Drawing for the job (mm, zero at the part's lowest x, y, z). Give positions to 0.01 mm unless a question says otherwise; leave off trailing zeros. Order: outer loops, then holes, each group sorted by start corner. A loop starts at its lowest first (then second) coordinate and runs counter-clockwise, first axis right, second up. Notation, with made-up numbers: (-21, -24.5) - (23, -24.5) arc R26 ccw to (23, 2.5) - close; hole circle Ø10 at (81, 19.5). An arc over 180 degrees is marked (long way). One line per item, written item: value.
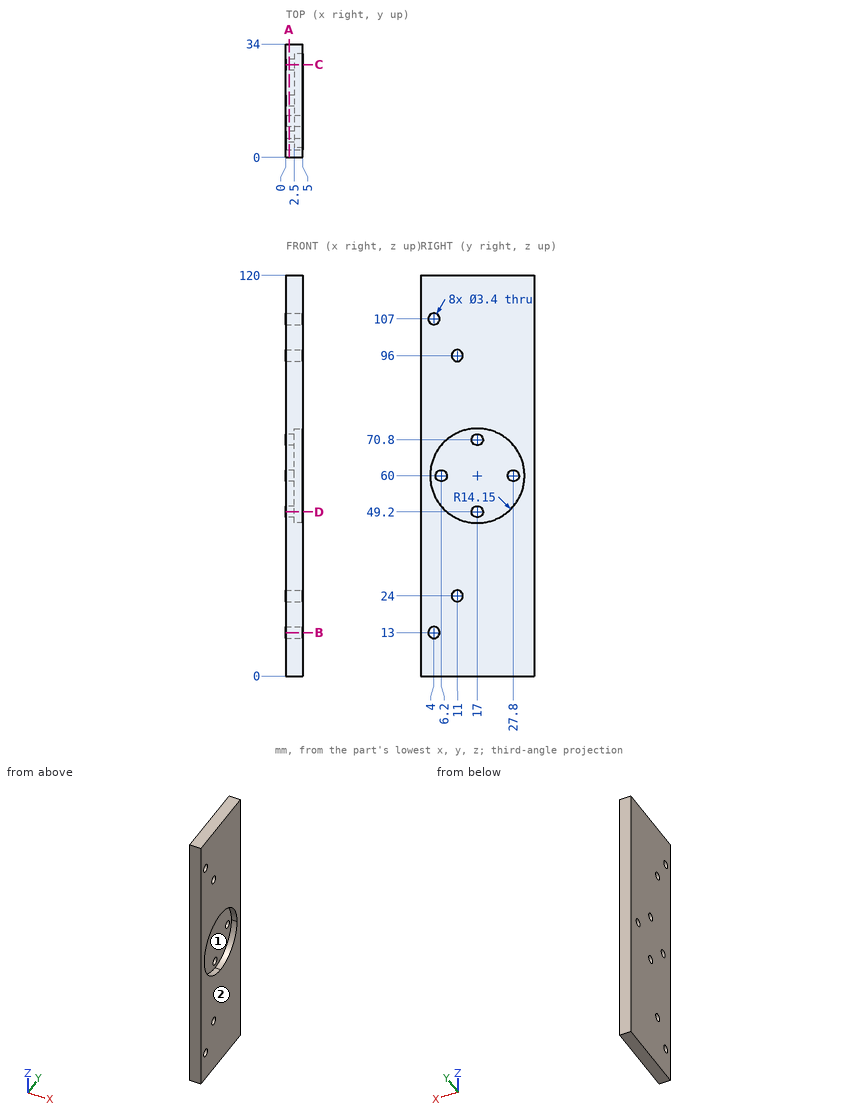
(1) Slice it at A-A, the plane x = 0.95. Count the separate pieces of the cut face and the enclosed holes in it, and give its area (3 significant figures).
Completed:
separate pieces: 1
enclosed holes: 8
area: 4,010 mm²
(2) Slice it at B-B, the plane z = 13. Give the cut face in (x, y).
Completed:
outline: (0, 0) - (5, 0) - (5, 2.3) - (0, 2.3) - close; (0, 5.7) - (5, 5.7) - (5, 34) - (0, 34) - close
(3) Pull direction Y, two halves, no side cores. Call the marked faces 1 and 2: +Y half, -Y half, draft (parallel to the pull), parting line (faces both ways), or undercut.
Completed:
face 1: undercut
face 2: draft
(4) Slice it at C-C, the plane y = 27.8. Give the cut face in (x, z).
Completed:
outline: (0, 0) - (5, 0) - (5, 50.86) - (2.5, 50.86) - (2.5, 58.3) - (0, 58.3) - close; (0, 61.7) - (2.5, 61.7) - (2.5, 69.14) - (5, 69.14) - (5, 120) - (0, 120) - close
(5) Slice it at D-D, the plane z = 49.2. Give the cut face in (x, y), and give its area (3 significant figures).
Completed:
outline: (0, 0) - (5, 0) - (5, 7.86) - (2.5, 7.86) - (2.5, 15.3) - (0, 15.3) - close; (0, 18.7) - (2.5, 18.7) - (2.5, 26.14) - (5, 26.14) - (5, 34) - (0, 34) - close
area: 116 mm²
(6) Pin check, flat tips, straight feed: P1, Ø2, axis at y = 13, z = 93, coming from the -X side; P2, Ø3, axis at y = 19.5, z = 68.5, coming from the +X side. Stop position of each tip, or through.
Completed:
P1: x = 0
P2: x = 2.5
(7) Drill centre lines: line 1 (Y direction, x = 2.35, z = 13); line 2 (Z direction, x = 3.25, y = 12); line 3 (Z direction, x = 3.8, y = 2.5). Where is each one in solid material? Low to high.
Completed:
line 1: 0 to 2.3, 5.7 to 34
line 2: 0 to 22.63, 25.37 to 46.76, 73.24 to 94.63, 97.37 to 120
line 3: 0 to 12.2, 13.8 to 106.2, 107.8 to 120
